Geometry: final body of the model. Coordinates: model frame, mm. A direction names the side the tool comes from. Round coordinates to 2 decimals unless told otherwise and drop trailing zeros. Loops run counter-clockwise (first coordinate to the right, second up) from the corner with the lowest first, then second, coordinate; pieces in that order, holes last. Notation, with made-up numbers: (71, -33) - (96, -33) arc R27 cw to (96, -4) - close; hole circle Ø6 at (23, 81.5). An arc over 180 degrees is marked (long way). Use CSV: the item, a comma, the result in double quotes.
from build123d import *

# Parameters (mm, degrees)
EXTRUDE_1_DEPTH = 10
FILLET_1_R      = 0.2


with BuildPart() as part:
    # Эскиз1 → Бобышка-Вытянуть1 (new body, symmetric)
    with BuildSketch(Plane.XY):
        Polygon((4, 0), (-4, 0), (-4, -3.3), (-9.75, -3.3), (-9.75, -5.8), (-4, -9.5), (4, -9.5), (9.75, -5.8), (9.75, -3.3), (4, -3.3), align=None)
    extrude(amount=EXTRUDE_1_DEPTH, both=True)

    # Эскиз4 → Отверстие обработанное метчиком M53 (revolve, cut)
    with BuildSketch(Plane(origin=(0, 0, 0), x_dir=(0, 0, 1), z_dir=(1, 0, 0))):
        Polygon((0, 0), (0, 9.5), (2.525, 9.5), (2.1, 9.075), (2.1, 0.425), (2.525, 0), align=None)
    revolve(axis=Axis((0, 6.35, 0), (0, -1, 0)), mode=Mode.SUBTRACT)

    # Скругление1
    fillet_1_edges = [part.edges().sort_by_distance(p)[0] for p in [
        (-4, 0, 0),
        (4, 0, 0),
        (4, -3.3, 0),
        (9.75, -3.3, 0),
        (4, -9.5, 0),
        (-4, -9.5, 0),
        (-9.75, -3.3, 0),
        (-4, -3.3, 0),
    ]]
    fillet(fillet_1_edges, radius=FILLET_1_R)


solid = part.part
Item 1: Section B-B on z = 0. Return the cut outline in (x, y) (3 decimals).
Final values:
outline,"(-9.75, -5.8) - (-4.049, -9.468) arc R0.2 ccw to (-3.941, -9.5) - (-2.525, -9.5) - (-2.1, -9.075) - (-2.1, -0.425) - (-2.525, 0) - (-3.8, 0) arc R0.2 ccw to (-4, -0.2) - (-4, -3.1) arc R0.2 cw to (-4.2, -3.3) - (-9.55, -3.3) arc R0.2 ccw to (-9.75, -3.5) - close; (2.1, -9.075) - (2.525, -9.5) - (3.941, -9.5) arc R0.2 ccw to (4.049, -9.468) - (9.75, -5.8) - (9.75, -3.5) arc R0.2 ccw to (9.55, -3.3) - (4.2, -3.3) arc R0.2 cw to (4, -3.1) - (4, -0.2) arc R0.2 ccw to (3.8, 0) - (2.525, 0) - (2.1, -0.425) - close"
Item 2: Section C-C on y = -4.75. Return the cut outline in (x, z).
Final values:
outline,"(-9.75, -10) - (9.75, -10) - (9.75, 10) - (-9.75, 10) - close; hole circle Ø4.2 at (0, 0)"
Item 3: Reachability of faces 1 (the flat face through (7, -3.3, 0)), 2 (the flat face through (-9.75, -5, 0)), 3 (the flat face through (-7, -3.3, 0)) from +Z, -Z, +X, -X, +Y, -Y: full face, straight path, thin tool, end or side. Return the list, or none.
Final values:
face 1,"+Z, -Z, +X, +Y"
face 2,"+Z, -Z, -X, +Y, -Y"
face 3,"+Z, -Z, -X, +Y"
Item 4: Mould query, pull axis Z, two halves, no side actions, for faces 4 (the cylindrical face through (-0.631, -4.689, 2.003)), 5 (the flat face through (0, -5, -10)), 6 (the flat face through (-4, -2, 0)). Classes: released by +Z, released by -Z, zero draft, split by the parting line, or undercut.
Final values:
face 4,"undercut"
face 5,"released by -Z"
face 6,"zero draft"
Item 5: Material intervals for line 1 (Z direction, x = 0, y = -7); line 2 (X direction, y = -2.75, z = 0); line 3 (X direction, y = -4, z = 0), sorted ascending.
Final values:
line 1,"z = -10 to -2.1, 2.1 to 10"
line 2,"x = -4 to -2.1, 2.1 to 4"
line 3,"x = -9.75 to -2.1, 2.1 to 9.75"
Item 6: Section D-D on z = -5. Return the cut outline in (x, y).
Final values:
outline,"(-9.75, -5.8) - (-4.05, -9.47) arc R0.2 ccw to (-3.94, -9.5) - (3.94, -9.5) arc R0.2 ccw to (4.05, -9.47) - (9.75, -5.8) - (9.75, -3.5) arc R0.2 ccw to (9.55, -3.3) - (4.2, -3.3) arc R0.2 cw to (4, -3.1) - (4, -0.2) arc R0.2 ccw to (3.8, 0) - (-3.8, 0) arc R0.2 ccw to (-4, -0.2) - (-4, -3.1) arc R0.2 cw to (-4.2, -3.3) - (-9.55, -3.3) arc R0.2 ccw to (-9.75, -3.5) - close"
Item 7: Pin query (flat end, axial travel): P1, Ø5, axis at x = 0, z = 0, coming from the +Y side (3 decimals); P2, Ø6, axis at x = -7, z = 5.5, coming from the -Y side; P3, Ø1.6, axis at x = 7, z = -2, coming from the +Y side. Return the tip coordinate at first contact, or that it passes through.
Final values:
P1,"stops at y = -0.025"
P2,"stops at y = -9.49"
P3,"stops at y = -3.3"
Item 8: Section A-A on x = 0. Return the cut outline in (y, z) (3 decimals).
Final values:
outline,"(-9.5, -10) - (0, -10) - (0, -2.525) - (-0.425, -2.1) - (-9.075, -2.1) - (-9.5, -2.525) - close; (-9.5, 2.525) - (-9.075, 2.1) - (-0.425, 2.1) - (0, 2.525) - (0, 10) - (-9.5, 10) - close"
